Verification items for the finished model (mm, model axes). A direction names the side the tool comes from. Round coordinates to 2 decimals unless told otherwise and drop trailing zeros. Order: outer loops, then holes, each group sorted by start corner. A loop starts at its lowest first (then second) coordinate and runs counter-clockwise, first axis right, second up.
```python
from build123d import *

# Parameters (mm, degrees)
F1_DEPTH       = 12.7
F3_DEPTH       = 6.35
F5_D           = 7.1374
F5_CSINK_D     = 13.4874
F5_CSINK_ANGLE = 82


with BuildPart() as f1:
    # F0 (on Top) → F1 (new body)
    with BuildSketch(Plane.XY):
        with BuildLine():
            Line((-76.2, 0), (-50.8, 0))
            ThreePointArc((-50.8, 0), (0, 50.8), (50.8, 0))
            Line((50.8, 0), (76.2, 0))
            ThreePointArc((76.2, 0), (0, 76.2), (-76.2, 0))
        make_face()
    extrude(amount=F1_DEPTH)

    # F2 (on face) → F3 (join)
    with BuildSketch(Plane(origin=(0, 0, 0), x_dir=(1, 0, 0), z_dir=(0, 0, -1))):
        with BuildLine():
            Line((-62.2170394667, -12.7), (-49.5170394667, -12.7))
            ThreePointArc((-49.5170394667, -12.7), (-62.2170394667, 0), (-74.9170394667, -12.7))
            Line((-74.9170394667, -12.7), (-62.2170394667, -12.7))
        make_face()
        with BuildLine():
            ThreePointArc((74.9170394667, -12.7), (62.2170394667, 0), (49.5170394667, -12.7))
            Line((49.5170394667, -12.7), (62.2170394667, -12.7))
            Line((62.2170394667, -12.7), (74.9170394667, -12.7))
        make_face()
    extrude(amount=F3_DEPTH)

    # F5 (through all)
    with Locations(Plane.XY.offset(12.7)):
        with Locations((-54.9926131403, 31.75), (-31.75, 54.9926131403), (0, 63.5), (31.75, 54.9926131403), (54.9926131403, 31.75)):
            CounterSinkHole(F5_D / 2, F5_CSINK_D / 2, counter_sink_angle=F5_CSINK_ANGLE)


solid = f1.part
```
1) Sectioned sample at A-A on x = 0. Record the cut outline in (y, z), then the cut area to 3 significant figures.
2) Sectioned sample at C-C on y = 31.75. Record the cut outline in (x, z).
3) Tool access check on faces 1 (the cylindrical face through (62, 0, -3)), 2 (the cylindrical face through (57.825, 29.579, 4.46)), 3 (the flat face through (62, 12.7, -3)). Record the directions out of +Z, -Z, +X, -X, +Y, -Y that give a thin tool (end or side, any length) a straight path to the whole face; none if there is none.
4) Draft check along X on faces 4 (the flat face through (-1, 56, 0)), 5 (the cylindrical face through (-62, 0, -3)), 6 (the cylindrical face through (1.68, 76.18, 6.26)). Enter one of: released by +X, released by -X, zero draft, split by the parting line, or undercut.
5) Sectioned sample at D-D on z = -3.75. Record the cut outline in (x, y).
6) Sectioned sample at B-B on y = 16. Record the cut outline in (x, z), then the cut area to 3 significant figures.
7) Scan lines: probe 1 along X at (y, z) = (31.75, 6); probe 2 along X at (y, z) = (35, 11.5); probe 3 along X at (y, z) = (52, 6.75). Record each from-to range of solid material in increasing order.
8) Go/stop test with flat-tipped pins: pin 1 Ø12 at (x, y) = (46, 24) entering from -Z; pin 2 Ø2 at (x, z) = (25.5, 8.5) entering from -Y; pin 3 Ø1 at (x, z) = (-19, 6) entering from -Y; pin 4 Ø4.5 at (x, y) = (31.75, 54.99) entering from +Z. Record where each tip stops, or that it passes through.
Returned:
1. outline: (50.8, 0) - (59.93, 0) - (59.93, 9.05) - (56.76, 12.7) - (50.8, 12.7) - close; (67.07, 0) - (76.2, 0) - (76.2, 12.7) - (70.24, 12.7) - (67.07, 9.05) - close
1. area: 220 mm2
2. outline: (-69.27, 0) - (-58.56, 0) - (-58.56, 9.05) - (-61.74, 12.7) - (-69.27, 12.7) - close; (-51.42, 0) - (-39.66, 0) - (-39.66, 12.7) - (-48.25, 12.7) - (-51.42, 9.05) - close; (39.66, 0) - (51.42, 0) - (51.42, 9.05) - (48.25, 12.7) - (39.66, 12.7) - close; (58.56, 0) - (69.27, 0) - (69.27, 12.7) - (61.74, 12.7) - (58.56, 9.05) - close
3. face 1: -Z, -Y
3. face 2: +Z, -Z
3. face 3: -Z, +X, -X, +Y
4. face 4: zero draft
4. face 5: undercut
4. face 6: split by the parting line
5. outline: (-74.92, 12.7) arc R12.7 ccw to (-49.52, 12.7) - close; (49.52, 12.7) arc R12.7 ccw to (74.92, 12.7) - close
6. outline: (-74.5, 0) - (-48.21, 0) - (-48.21, 12.7) - (-74.5, 12.7) - close; (48.21, 0) - (74.5, 0) - (74.5, 12.7) - (48.21, 12.7) - close
6. area: 668 mm2
7. probe 1: x = -69.27 to -58.56, -51.42 to -39.66, 39.66 to 51.42, 58.56 to 69.27
7. probe 2: x = -67.69 to -59.68, -50.31 to -36.82, 36.82 to 50.31, 59.68 to 67.69
7. probe 3: x = -55.7 to -33.69, -29.81 to 29.81, 33.69 to 55.7
8. pin 1: stops at z = 0
8. pin 2: stops at y = 43.34
8. pin 3: stops at y = 46.91
8. pin 4: passes through
